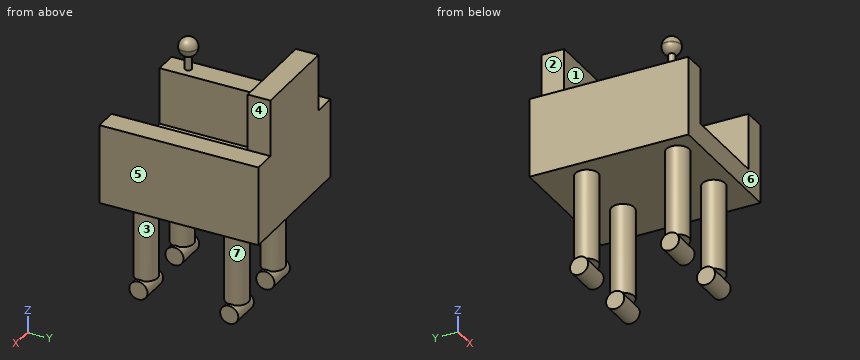
from build123d import *

# Parameters (mm, degrees)
F0_W      = 127
F0_H      = 25.4
F1_DEPTH  = 76.2
F2_R      = 12.7
F3_DEPTH  = 101.6
F5_START  = 20.32
F4_R      = 10.16
F5_DEPTH  = 33.02
F6_START  = 43.18
F5_FACE_R = 10.16
F6_DEPTH  = 33.02
F7_DEPTH  = 25.4
F8_W      = 25.4
F8_H      = 152.4
F9_DEPTH  = 63.5
F10_DEPTH = 25.4
F11_W     = 101.6
F11_H     = 25.4
F12_DEPTH = 127
F13_R     = 3.81
F14_DEPTH = 25.4
F15_R     = 10.16
F16_DEPTH = 10.16


# Not quite as in the source:
# - a fillet or chamfer that OpenCascade refuses, or shapes differently, is made with other operations: its cross-section is extruded or revolved along the edge and cut away or added


with BuildPart() as f1:
    # F0 (on Front) → F1 (new body, symmetric)
    with BuildSketch(Plane.XZ):
        with Locations((-1.2627113611, -2.0410835827)):
            Rectangle(F0_W, F0_H)
    extrude(amount=F1_DEPTH, both=True)

    # F2 (on face) → F3 (join)
    with BuildSketch(Plane(origin=(0, 0, -14.7410835827), x_dir=(1, 0, 0), z_dir=(0, 0, -1))):
        with Locations((-39.3627113611, 50.8)):
            Circle(F2_R)
        with Locations((36.8372886389, 50.8)):
            Circle(F2_R)
        with Locations((36.8372886389, -50.8)):
            Circle(F2_R)
        with Locations((-39.3627113611, -50.8)):
            Circle(F2_R)
    extrude(amount=F3_DEPTH)

    # F4 (on Right) → F5 (join)
    with BuildSketch(Plane.YZ.offset(F5_START)):
        with Locations((-50.8, -125.73)):
            Circle(F4_R)
        with Locations((50.8, -125.73)):
            Circle(F4_R)
    extrude(amount=F5_DEPTH)

    # F5_face (on face) → F6 (join)
    with BuildSketch(Plane(origin=(20.32, 50.8, -125.73), x_dir=(0, 1, 0), z_dir=(-1, 0, 0)).offset(F6_START)):
        Circle(F5_FACE_R)
        with Locations((-101.6, 0)):
            Circle(F5_FACE_R)
    extrude(amount=F6_DEPTH)

    # F7 (add): a face of the model
    f7_faces = [f1.faces().sort_by_distance(p)[0] for p in [
        (62.2372886389, 0, -2.0410835827),
    ]]
    extrude(f7_faces, amount=F7_DEPTH)

    # F8 (on face) → F9 (join)
    with BuildSketch(Plane.XY.offset(10.6589164173)):
        with Locations((74.9372886389, 0)):
            Rectangle(F8_W, F8_H)
        with Locations((-52.0627113611, 0)):
            Rectangle(F8_W, F8_H)
    extrude(amount=F9_DEPTH)

    # F10 (add): a face of the model
    f10_faces = [f1.faces().sort_by_distance(p)[0] for p in [
        (11.4372886389, 76.2, 8.8945760307),
    ]]
    extrude(f10_faces, amount=F10_DEPTH)

    # F11 (on face) → F12 (join)
    with BuildSketch(Plane.XY.offset(10.6589164173)):
        with Locations((11.4372886389, 88.9)):
            Rectangle(F11_W, F11_H)
    extrude(amount=F12_DEPTH)

    # F13 (on face) → F14 (join)
    with BuildSketch(Plane.XY.offset(74.1589164173)):
        with Locations((-52.0627113611, -50.8)):
            Circle(F13_R)
    extrude(amount=F14_DEPTH)

    # F15 (on face) → F16 (join, symmetric)
    with BuildSketch(Plane.XY.offset(99.5589164173)):
        with Locations((-52.0627113611, -50.8)):
            Circle(F15_R)
    extrude(amount=F16_DEPTH, both=True)

    # F17: fillet of radius 10.159746 on 2 edges, made by hand

    # F17_s1 → F17_t2 (revolve, cut)
    with BuildSketch(Plane.XZ.offset(50.8)):
        with BuildLine():
            ThreePointArc((-41.9027113611, 99.5591704173), (-44.8784320693, 106.7431957091), (-52.0624573611, 109.7189164173))
            Line((-52.0624573611, 109.7189164173), (-41.9027113611, 109.7189164173))
            Line((-41.9027113611, 109.7189164173), (-41.9027113611, 99.5591704173))
        make_face()
    revolve(axis=Axis((-52.0627113611, -50.8, 109.7189164173), (0, 0, 1)), mode=Mode.SUBTRACT)

    # F17_s3 → F17_t4 (revolve, cut)
    with BuildSketch(Plane.XZ.offset(50.8)):
        with BuildLine():
            ThreePointArc((-48.2527113611, 89.3989164173), (-43.6384888643, 93.1377755804), (-41.9027113611, 98.8173172476))
            Line((-41.9027113611, 98.8173172476), (-41.9027113611, 89.3989164173))
            Line((-41.9027113611, 89.3989164173), (-48.2527113611, 89.3989164173))
        make_face()
    revolve(axis=Axis((-52.0627113611, -50.8, 89.3989164173), (0, 0, 1)), mode=Mode.SUBTRACT)


solid = f1.part
Could you check a few things on this model? Use its own coordinates, in mm. Face numbers are marked on the shaded views. A direction names the side the tool comes from. Round coordinates to 2 decimals unless told otherwise and drop trailing zeros. Order: outer loops, then holes, each group sorted by start corner. A loop starts at its lowest first (then second) coordinate and runs counter-clockwise, first axis right, second up.
Q1. Imagine slicing it at B-B, the plane y = -15.5. List the corners of the cut face in (x, z) for me.
Geometry says:
outline: (-64.76, -14.74) - (87.64, -14.74) - (87.64, 74.16) - (62.24, 74.16) - (62.24, 10.66) - (-39.36, 10.66) - (-39.36, 74.16) - (-64.76, 74.16) - close
Q2. Imagine slicing it at A-A, the plane z = -125.73. List the corners of the cut face in (x, y) for me, then the cut area to 3 significant figures.
Geometry says:
outline: (-55.88, -60.96) - (-22.86, -60.96) - (-22.86, -40.64) - (-55.88, -40.64) - close; (-55.88, 40.64) - (-22.86, 40.64) - (-22.86, 60.96) - (-55.88, 60.96) - close; (20.32, -60.96) - (53.34, -60.96) - (53.34, -40.64) - (20.32, -40.64) - close; (20.32, 40.64) - (53.34, 40.64) - (53.34, 60.96) - (20.32, 60.96) - close
area: 2,680 mm2
Q3. Imagine slicing it at C-C, the plane x = 67. List the corners of the cut face in (y, z) for me.
Geometry says:
outline: (-76.2, -14.74) - (101.6, -14.74) - (101.6, 74.16) - (-76.2, 74.16) - close
Q4. I'm going to push flat-ended pins straight in: P1, Ø5, axis at x = 6.5, y = -52.5, coming from the +Z side; P2, Ø6, axis at y = -48, z = -126, coming from the -X side; P3, Ø9.5, axis at x = 40.5, y = 44.5, coming from the -Z side; P4, Ø12, axis at x = 14, z = -33, coming from the -Y side. Where does each tip first touch, or does it pass through?
Geometry says:
P1: stops at z = 10.66
P2: stops at x = -55.88
P3: stops at z = -135.77
P4: passes through
Q5. Please list where these lines run through material, in increasing order: probe 1 along X at (y, z) = (-38, 15); probe 2 along Y at (x, z) = (47, 74.5); probe 3 along Z at (x, y) = (53, -66).
Geometry says:
probe 1: x = -64.76 to -39.36, 62.24 to 87.64
probe 2: y = 76.2 to 101.6
probe 3: z = -14.74 to 10.66
Q6. Which directions (+Z, -Z, +X, -X, +Y, -Y) give clear straight access to the entire face, cutting with the end or side of a thin tool? Please do the marked faces 1, 2, 3 and 4.
Geometry says:
face 1: +Z, -Y
face 2: +Z, -X, +Y, -Y
face 3: none
face 4: +Z, +X, +Y, -Y
Q7. Imagine slicing it at D-D, the plane y = 50.8. List the corners of the cut face in (x, z) for me.
Geometry says:
outline: (-64.76, -14.74) - (-52.06, -14.74) - (-52.06, -115.57) - (-55.88, -115.57) - (-55.88, -135.89) - (-22.86, -135.89) - (-22.86, -115.57) - (-26.66, -115.57) - (-26.66, -14.74) - (24.14, -14.74) - (24.14, -115.57) - (20.32, -115.57) - (20.32, -135.89) - (53.34, -135.89) - (53.34, -115.57) - (49.54, -115.57) - (49.54, -14.74) - (87.64, -14.74) - (87.64, 74.16) - (62.24, 74.16) - (62.24, 10.66) - (-39.36, 10.66) - (-39.36, 74.16) - (-64.76, 74.16) - close
Q8. Thinking about a two-plate mould opening in Y: for the marked faces 5, 6 and 7, which applies, released by +Y, released by -Y, zero draft, split by the parting line, or undercut?
Geometry says:
face 5: zero draft
face 6: released by -Y
face 7: undercut
